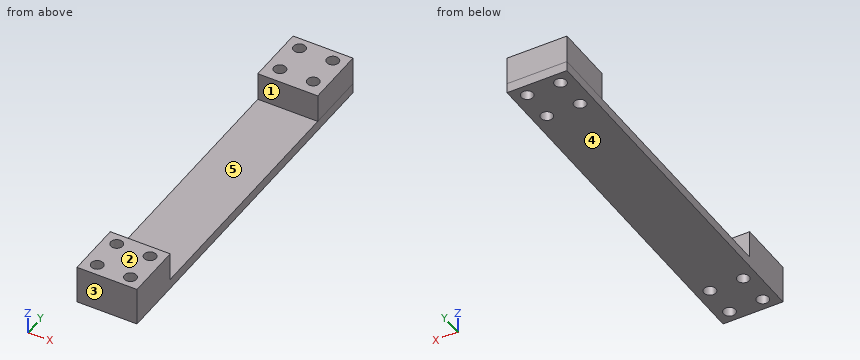
```python
from build123d import *

# Parameters (mm, degrees)
SKETCH2_W            = 18
SKETCH2_H            = 110.4
BOSS_EXTRUDE1_DEPTH  = 3
BOSS_EXTRUDE2_DEPTH  = 8.50551692
M3_CLEARANCE_HOLE1_D = 3.6


with BuildPart() as part:
    # Sketch2 → Boss-Extrude1 (new body)
    with BuildSketch(Plane.XY.offset(-0.25)):
        with Locations((5.631550422, -23.757430205)):
            Rectangle(SKETCH2_W, SKETCH2_H)
    extrude(amount=-BOSS_EXTRUDE1_DEPTH)

    # Sketch3 → Boss-Extrude2 (add)
    with BuildSketch(Plane.XY.offset(-0.25)):
        Polygon((-3.368449578, 31.442569795), (14.631550422, 31.442569738), (14.631550364, 13.442569738), (-3.368449636, 13.442569795), align=None)
        Polygon((-3.368449578, -61.957430205), (14.631550422, -61.957430262), (14.631550422, -78.957430205), (-3.368449578, -78.957430205), align=None)
    extrude(amount=BOSS_EXTRUDE2_DEPTH)

    # M3 Clearance Hole1 (through all)
    with Locations(Plane.XY.offset(8.25551692)):
        with Locations((0.631550422, -65.457430205), (0.631550422, -75.457430205), (10.631550422, -75.457430205), (10.631550422, -65.457430205), (0.631550422, 17.942569795), (10.631550422, 17.942569795), (10.631550422, 27.942569795), (0.631550422, 27.942569795)):
            Hole(M3_CLEARANCE_HOLE1_D / 2)


solid = part.part
```
Design review of the part built by this model. Coordinates are the model's own, in mm. Face numbers are marked on the shaded views. A direction names the side the tool comes from. Give positions to 0.01 mm unless a question says otherwise; leave off trailing zeros. Write each loop counter-clockwise with the first axis right and the second up, starting at its lowest first coordinate (ties: lowest second). Pieces come first, ordered by that corner, then holes. Notation, with made-up numbers: (83, -22) -> (89, -22) arc R18 ccw to (89, -9) -> close; hole circle Ø11 at (85, -32.5). An arc over 180 degrees is marked (long way). Answer in a Markdown table with one row per item.
(1) Consider section B-B (x = 6). State the section outline as (y, z) points, then the cut area to 3 significant figures.
Results:
| item | result |
|---|---|
| outline | (-78.96, -3.25) -> (31.44, -3.25) -> (31.44, 8.26) -> (13.44, 8.26) -> (13.44, -0.25) -> (-61.96, -0.25) -> (-61.96, 8.26) -> (-78.96, 8.26) -> close |
| area | 629 mm2 |
(2) Mouldability with a two-part tool opening along Y and no side actions: class the marked faces 1, 2 and 3 as +Y half, -Y half, draft (parallel to the pull), parting line (faces both ways), or undercut.
Results:
| item | result |
|---|---|
| face 1 | undercut |
| face 2 | draft |
| face 3 | -Y half |
(3) Clearance check with flat-ended pins moving along their axes: pin 1 (2 mm diameter, centred on x = 10.5, y = -5, fed in from +Z); pin 2 (3 mm diameter, centred on x = 0.63, y = 17.94, fed in from -Z). State where each tip first meets the part, or that it passes through.
Results:
| item | result |
|---|---|
| pin 1 | z = -0.25 |
| pin 2 | through |
(4) Consider section A-A (z = 7). Count the separate pieces of the cut face and the enclosed holes in it, then the cut area to 3 significant figures.
Results:
| item | result |
|---|---|
| separate pieces | 2 |
| enclosed holes | 8 |
| area | 549 mm2 |
(5) To check wall thickness, follow probe 1 along Y at (x, z) = (10.5, 0.5); probe 2 along Y at (x, z) = (6.5, 1.5); probe 3 along Y at (x, z) = (9.5, 4.5). State the ranges of each line that lie inside material, in increasing order.
Results:
| item | result |
|---|---|
| probe 1 | -78.96 to -77.25, -73.66 to -67.25, -63.66 to -61.96, 13.44 to 16.15, 19.74 to 26.15, 29.74 to 31.44 |
| probe 2 | -78.96 to -61.96, 13.44 to 31.44 |
| probe 3 | -78.96 to -76.86, -74.06 to -66.86, -64.06 to -61.96, 13.44 to 16.54, 19.34 to 26.54, 29.34 to 31.44 |
(6) For the marked faces 4 and 5, list the 3-axis set-ups (+Z, -Z, +X, -X, +Y, -Y) from which the entire face can be reached by the end or side of a thin tool; tool diameter is ignored.
Results:
| item | result |
|---|---|
| face 4 | -Z, +X, -X, +Y, -Y |
| face 5 | +Z, +X, -X |
(7) Consider section D-D (y = -36). State the section outline as (x, z) points, then the cut area to 3 significant figures.
Results:
| item | result |
|---|---|
| outline | (-3.37, -3.25) -> (14.63, -3.25) -> (14.63, -0.25) -> (-3.37, -0.25) -> close |
| area | 54.0 mm2 |
